Solid Edge part; units mm, degrees
sketch "Sketch1" plane through (0, 0, 0) normal (1, 0, 0) x (0, 1, 0)
  circle A0 centre (-77.515, 0) radius 2.4892
  arc A1 (-74.0618, -0.5) -> (-74.0618, 0.5) centre (-77.515, 0) cw
  line L0 (-74.0618, -0.5) -> (74.0618, -0.5)
  arc A2 (74.0618, -0.5) -> (74.0618, 0.5) centre (77.515, 0) ccw
  line L1 (-74.0618, 0.5) -> (74.0618, 0.5)
  circle A3 centre (77.515, 0) radius 2.4892
extrude "Protrusion1" add sketch "Sketch1" along normal mid plane 50
properties material "Nylon, general purpose"
Geometry: final body of the model. Coordinates: model frame, mm. A direction names the side the tool comes from. Coordinates: 2 decimals unless noted, no trailing zeros. Order: outer loops, then holes, each group sorted by start corner. A loop starts at its lowest first (then second) coordinate and runs counter-clockwise, first axis right, second up. Notation, with made-up numbers: (-20.75, -21.75) -> (-15.75, -21.75) arc R20 cw to (-15.75, -12.75) -> close; hole circle Ø1 at (-2, -30.75). An arc over 180 degrees is marked (long way). Use CSV: the item, a comma, the result in double quotes.
1) Line query: line 1 (Y direction, x = -20.5, z = -1.5); line 2 (Z direction, x = 10.5, y = -51); line 3 (Y direction, x = -18, z = 2). Output: solid intervals per line, ascending.
Findings:
line 1,"y = -80.67 to -79.5, -75.53 to -74.36, 74.36 to 75.53, 79.5 to 80.67"
line 2,"z = -0.5 to 0.5"
line 3,"y = -80.37 to -79, -76.03 to -74.66, 74.66 to 76.03, 79 to 80.37"
2) Mould query, pull axis Z, two halves, no side actions, for faces 1 (the flat face through (25, 0, 0)), 2 (the cylindrical face through (-0.35, -81, -0.15)), 3 (the cylindrical face through (-0.35, -80, -0.11)). Classes: +Z half, -Z half, draft (parallel to the pull), parting line (faces both ways), or undercut.
Findings:
face 1,"draft"
face 2,"parting line"
face 3,"undercut"
3) Section A-A on x = 15. Output: boundary loops of the cut face in (y, z) (3 decimals), then the cut area to 3 significant figures.
Findings:
outline,"(-74.062, -0.5) -> (74.062, -0.5) arc R3.489 ccw (long way) to (74.062, 0.5) -> (-74.062, 0.5) arc R3.489 ccw (long way) to start; hole circle Ø4.978 at (-77.515, 0); hole circle Ø4.978 at (77.515, 0)"
area,"186 mm^2"
4) Section B-B on y = -52. Output: boundary loops of the cut face in (x, z).
Findings:
outline,"(-25, -0.5) -> (25, -0.5) -> (25, 0.5) -> (-25, 0.5) -> close"
5) Pin query (flat end, axial travel): pin 1 Ø15 at (x, y) = (-3.5, 11) entering from +Z; pin 2 Ø10 at (x, y) = (-16.5, 10.5) entering from -Z. Return the tip coordinate at first contact, or that it passes through.
Findings:
pin 1,"stops at z = 0.5"
pin 2,"stops at z = -0.5"
6) Access query for faces 4 (the cylindrical face through (-0.35, 79.814, 0.953)), 5 (the flat face through (0, -1, 0.5)), 6 (the flat face through (0, -1, -0.5)). Directions: +Z, -Z, +X, -X, +Y, -Y. A direction counts if a zero-diameter tool reaches every point of the face in a straight line with its end or side. Return the directions, or none.
Findings:
face 4,"+X, -X"
face 5,"+Z, +X, -X"
face 6,"-Z, +X, -X"
